Read the model definition and answer for the solid it produces. Units are mm, in the model's axes. Round coordinates to 2 decimals unless told otherwise and drop trailing zeros. Write each loop counter-clockwise with the first axis right and the second up, starting at its lowest first coordinate (ties: lowest second). Pieces come first, ordered by that corner, then holes. Notation, with made-up numbers: (80.25, 8) -> (118.25, 8) arc R12 cw to (118.25, 16) -> close; hole circle Ø11 at (72.25, 57). An arc over 180 degrees is marked (long way). Return JSON: item names as keys, results as strings. Group by question number.
(1) A cutting plane is placed at A-A on z = 17. Give the vertices of the cut face in (x, y).
(2) A cutting plane is placed at B-B on x = 9.5. Give the vertices of the cut face in (y, z).
(3) Straight lines are drawn through the part: line 1 (X direction, y = -354, z = 22); line 2 (X direction, y = -820.5, z = 19); line 3 (Y direction, x = 179.5, z = 7). For each, find the intervals that lie inside material, in ascending order.
(4) A cutting plane is placed at C-C on y = -801. Give the vertices of the cut face in (x, z), then the cut area to 3 significant figures.
(5) Given pin 1 (1.5 mm diameter, centred on x = 303, z = 22.5, fed in from -Y); pin 2 (5 mm diameter, centred on y = -1336, z = 28, fed in from +X); pin 3 (5 mm diameter, centred on x = 261, z = 21, fed in from -Y), each flat-ended and moving along its own axis, determine where each tip first touches the part or whether it passes through.
Autodesk Inventor part; units mm, degrees
ref_plane "YZ Plane" through (0, 0, 0) normal (1, 0, 0) x (0, 1, 0)
ref_plane "XZ Plane" through (0, 0, 0) normal (0, 1, 0) x (-1, 0, 0)
ref_plane "XY Plane" through (0, 0, 0) normal (0, 0, 1) x (1, 0, 0)
sketch "Sketch1" plane through (0, 0, 0) normal (0, 0, 1) x (1, 0, 0)
  line L0 (-571.5, -1549.4) -> (571.5, -1549.4)
  line L1 (571.5, -1549.4) -> (571.5, 1549.4)
  line L2 (571.5, 1549.4) -> (-571.5, 1549.4)
  line L3 (-571.5, 1549.4) -> (-571.5, -1549.4)
  line L4 (-571.5, -1549.4) -> (571.5, 1549.4) construction
  line L5 (571.5, -1549.4) -> (-571.5, 1549.4) construction
  line L6 (-571.5, 0) -> (571.5, 0)
  line L7 (571.5, 0) -> (-571.5, -1549.4)
  line L8 (-535.73, -1575.7877) -> (-607.27, -1523.0123)
  line L9 (607.27, -26.3877) -> (535.73, 26.3877)
  line L10 (535.73, 26.3877) -> (-607.27, -1523.0123)
  line L11 (-535.73, -1575.7877) -> (607.27, -26.3877)
  line L12 (535.73, 26.3877) -> (571.5, 74.8759)
  line L13 (-571.5, 1549.4) -> (571.5, -1549.4) construction
  line L14 (571.5, 0) -> (-571.5, 1549.4)
  line L15 (-535.73, 1575.7877) -> (-607.27, 1523.0123)
  line L16 (607.27, 26.3877) -> (535.73, -26.3877)
  line L17 (535.73, -26.3877) -> (-607.27, 1523.0123)
  line L18 (-535.73, 1575.7877) -> (607.27, 26.3877)
  line L19 (535.73, -26.3877) -> (571.5, -74.8759)
  point P0 (0, 0)
  point P1 (571.5, 74.8759)
  point P2 (-516.2637, 1549.4)
  point P3 (-571.5, 1474.5241)
  point P4 (571.5, -74.8759)
  point P5 (571.5, -74.8759)
  point P6 (516.2637, 0)
  point P7 (-571.5, -1474.5241)
  point P8 (-516.2637, -1549.4)
  dimension "d0" = 1143
  dimension "d1" = 3098.8
  dimension "d3" = 88.9
  dimension "d4" = 88.9
extrude "Extrusion1" add sketch "Sketch1" along normal blind 38.1 contours L7 L19 L11 L0 | L3 L10 L17 L19 L7
properties part number "74+"
Checks:
{
 "1": {"outline": "(-571.5, -1549.4) -> (-516.26, -1549.4) -> (571.5, -74.88) -> (535.73, -26.39) -> (516.26, 0) -> (-571.5, -1474.52) -> close"},
 "2": {"outline": "(-836.7, 0) -> (-686.95, 0) -> (-686.95, 38.1) -> (-836.7, 38.1) -> close"},
 "3": {"line 1": "x = 255.12 to 365.59", "line 2": "x = -89.02 to 21.45", "line 3": "y = -606.25 to -456.5"},
 "4": {"outline": "(-74.64, 0) -> (35.83, 0) -> (35.83, 38.1) -> (-74.64, 38.1) -> close", "area": "4,210 mm^2"},
 "5": {"pin 1": "stops at y = -439.86", "pin 2": "stops at x = -356.99", "pin 3": "stops at y = -499.16"}
}
